```python
from build123d import *


with BuildPart() as part:
    # Sketch1 → Revolve7 (revolve)
    with BuildSketch(Plane.XY):
        with BuildLine():
            Line((-53.975, 0), (-53.975, 25.4))
            Line((-53.975, 25.4), (-60.325, 25.4))
            Line((-60.325, 25.4), (-60.325, 38.1))
            Line((-60.325, 38.1), (-54.876478898, 38.1))
            ThreePointArc((-54.876478898, 38.1), (-52.968691921, 38.737092624), (-51.826534557, 40.392693639))
            ThreePointArc((-51.826534557, 40.392693639), (-34.904240815, 66.539573647), (-6.35, 78.976562476))
            Line((-6.35, 78.976562476), (-6.35, 75.801562476))
            ThreePointArc((-6.35, 75.801562476), (-38.1, 59.001041651), (-50.8, 25.4))
            Line((-50.8, 25.4), (-50.8, 0))
            Line((-50.8, 0), (-53.975, 0))
        make_face()
    revolve(axis=Axis((0, 121.236821391, 0), (0, -1, 0)))


solid = part.part
```
Model file for the job. Use its own axes, mm. A direction names the side the tool comes from. Give positions to 0.01 mm unless a question says otherwise; leave off trailing zeros. Loops run counter-clockwise (first coordinate to the right, second up) from the corner with the lowest first, then second, coordinate; pieces in that order, holes last. Notation, with made-up numbers: (57, -33) -> (100, -33) arc R27 cw to (100, -4) -> close; hole circle Ø8 at (50, -5). An arc over 180 degrees is marked (long way). Use CSV: the item, a comma, the result in double quotes. Start each with the question number.
1) Tool access for faces 1 (the cylindrical face through (39.78, 12.88, -36.48)), 2 (the flat face through (40, 0, 32)): list every direction of +Z, -Z, +X, -X, +Y, -Y with a clear straight run to the whole face (end or side of a thin tool).
2) Slice it at C-C on y = 32. Give the cut face in (x, z) (3 decimals).
3) Slice it at A-A on z = 0. Give the cut face in (x, y) (3 decimals), plus the area to 3 significant figures.
4) Mould opens along X. For faces 3 (the cylindrical face through (60.267, 31.839, -2.652)), 4 (the cylindrical face through (1.38, 77.37, 6.2)), 5 (the flat face through (13.7, 38.1, 53.3)), 6 (the cylindrical face through (11.012, 12.522, 49.592)) say: released by +X, released by -X, zero draft, split by the parting line, or undercut.
5) Wall check: line 1 (X direction, y = 13.5, z = 0) (3 decimals); line 2 (Y direction, x = 36.5, z = 46). Give the ranges that are in metal, low to high.
6) Slice it at B-B on x = 0. Give the cut face in (y, z) (3 decimals).
7) Flat gauge pins, fed straight in: pin 1 Ø5 at (x, z) = (15.5, 27) entering from +Y; pin 2 Ø3 at (x, y) = (10, 12) entering from +Z; pin 3 Ø3 at (y, z) = (48, 22.5) entering from +X. Where does each tip first touch, or does it go through?
Computed values:
1,face 1,"-Y"
1,face 2,"+Z, -Z, +X, -X, -Y"
2,outline,"circle Ø120.65 at (0, 0); hole circle Ø100.739 at (0, 0)"
3,outline,"(-60.325, 25.4) -> (-53.975, 25.4) -> (-53.975, 0) -> (-50.8, 0) -> (-50.8, 25.4) arc R50.8 cw to (-6.35, 75.802) -> (-6.35, 78.977) arc R53.952 ccw to (-51.827, 40.393) arc R3.175 cw to (-54.876, 38.1) -> (-60.325, 38.1) -> close; (6.35, 75.802) arc R50.8 cw to (50.8, 25.4) -> (50.8, 0) -> (53.975, 0) -> (53.975, 25.4) -> (60.325, 25.4) -> (60.325, 38.1) -> (54.876, 38.1) arc R3.175 cw to (51.827, 40.393) arc R53.952 ccw to (6.35, 78.977) -> close"
3,area,"817 mm^2"
4,face 3,"split by the parting line"
4,face 4,"undercut"
4,face 5,"zero draft"
4,face 6,"undercut"
5,line 1,"x = -53.975 to -50.8, 50.8 to 53.975"
5,line 2,"y = 25.4 to 38.1"
6,outline,"(0, -53.975) -> (25.4, -53.975) -> (25.4, -60.325) -> (38.1, -60.325) -> (38.1, -54.876) arc R3.175 cw to (40.393, -51.827) arc R53.952 ccw to (78.977, -6.35) -> (75.802, -6.35) arc R50.8 cw to (25.4, -50.8) -> (0, -50.8) -> close; (0, 50.8) -> (25.4, 50.8) arc R50.8 cw to (75.802, 6.35) -> (78.977, 6.35) arc R53.952 ccw to (40.393, 51.827) arc R3.175 cw to (38.1, 54.876) -> (38.1, 60.325) -> (25.4, 60.325) -> (25.4, 53.975) -> (0, 53.975) -> close"
7,pin 1,"stops at y = 71.13"
7,pin 2,"stops at z = 53.3"
7,pin 3,"stops at x = 44.58"
